Here's how the part is built. I have some questions about the finished solid (model axes, mm). Face numbers are marked on the shaded views. A direction names the side the tool comes from. Coordinates: 2 decimals unless noted, no trailing zeros. Write each loop counter-clockwise with the first axis right and the second up, starting at its lowest first coordinate (ties: lowest second). Pieces come first, ordered by that corner, then holes.
Item 1: For the marked faces 1 and 2, which set-ups out of +Z, -Z, +X, -X, +Y, -Y let a thin tool reach every point of the face, with its end or its side?
Item 2: If I drill on line 1 (Z direction, x = -0.05, y = -0.2); line 2 (Z direction, x = -0.85, y = -0.7); line 3 (X direction, y = -0.05, z = -7.75), over which ranges is the centre line in solid material (lowest first)?
Item 3: If we section it at A-A (z = -4.5): Please give me the cut outline in (x, y), then the cut area to 3 significant figures.
Item 4: I'm going to push flat-ended pins straight in: pin 1 Ø0.9 at (x, z) = (-0.5, -0.5) entering from -Y; pin 2 Ø0.9 at (x, z) = (0.5, -1) entering from -Y; pin 3 Ø1.3 at (y, z) = (1, -0.5) entering from -X; pin 4 Ø1.5 at (x, z) = (0.5, -6.5) entering from +Y. Where does each tip first touch, or does it pass through?
Autodesk Inventor part; units mm, degrees
ref_plane "MSC_PF1" through (0, 0, 0) normal (1, 0, 0) x (0, 1, 0)
ref_plane "MSC_PT1" through (0, 0, 0) normal (0, 0, -1) x (-1, 0, 0)
ref_plane "YZ Plane" through (0, 0, 0) normal (1, 0, 0) x (0, 1, 0)
sketch "Skizze1" plane through (0, 0, 0) normal (0, 1, 0) x (-1, 0, 0)
  point P0 (0, 0)
sketch "Skizze2" plane through (0, 0, 0) normal (0, 0, 1) x (1, 0, 0)
  point P0 (0, 0)
sketch "Skizze3" plane through (0, 0, 0) normal (0, 1, 0) x (-1, 0, 0)
  line L0 (-2.35, 0) -> (0, 0)
  line L1 (-2.35, -0.4) -> (-2.35, 0)
  line L2 (-1.25, -1.5) -> (-2.35, -0.4)
  line L3 (-1.25, -1.95) -> (-1.25, -1.5)
  line L4 (-1.025, -2.175) -> (-1.25, -1.95)
  line L5 (-1.25, -2.625) -> (-1.025, -2.175)
  line L6 (-1.25, -10) -> (-1.25, -2.625)
  line L7 (0, 0) -> (0, -10)
  line L8 (0, 3.3392) -> (0, -10.6608) construction
  line L9 (0, 3.3392) -> (0, -10.6608)
  line L10 (0, -13.4608) -> (0, 6.1392)
  line L11 (-1.25, -10) -> (0, -10)
  line L12 (0.47, 0) -> (-2.82, 0)
  dimension "d3" = 2.35
  dimension "d5" = 0.45
  dimension "d7" = 0.225
  dimension "d9" = 0.45
  dimension "d11" = 1.5
  dimension "d13" = 135
  dimension "d15" = 10
  dimension "d17" = 1.025
  dimension "d19" = 0
  dimension "d41" = 1.25
revolve "Drehung1" add sketch "Skizze3" angle 360 about axis through (0, 0, 3.3392) along (0, 0, -1)
sketch "Skizze4" plane through (0, 0, 0) normal (0, 1, 0) x (-1, 0, 0)
  line L0 (-1.4, 0) -> (0, 0)
  line L1 (-0.2333, -1.3636) -> (-1.4, 0)
  line L2 (0, -1.3636) -> (-0.2333, -1.3636)
  line L3 (0, 0) -> (0, -1.3636)
  line L4 (-1.25, -1.5) -> (1.25, -1.5) construction
  line L5 (-2.35, 0) -> (2.35, 0)
  line L6 (0, -1.8) -> (0, 0.3)
  dimension "d22" = 1.4
  dimension "d24" = 0.2333
  dimension "d26" = 1.3636
extrude "Extrusion1" cut sketch "Skizze4" along normal mid plane 0.4667
pattern_circular "Polare Anordnung1" count 4 over 360 about axis through (0, 0, 0) along (0, 0, 1) of "Extrusion1"
thread "Gewinde1"
ref_plane "MSC_PF1" through (0, 0, 0) normal (1, 0, 0) x (0, 1, 0)
ref_plane "MSC_PT1" through (0, 0, 0) normal (0, 0, -1) x (-1, 0, 0)
equation "\"d3\" = 0.5 * Dh"
equation "\"d5\" = msp_x"
equation "\"d7\" = ParA"
equation "\"d9\" = msp_x"
equation "\"d11\" = ParK"
equation "\"d15\" = NLG"
equation "\"d17\" = 0.5 * msp_mdtds"
equation "\"d41\" = 0.5 * NND"
equation "\"d22\" = 0.5 * M"
equation "\"d24\" = 0.0833333 * M"
equation "\"d26\" = 0.909091 * ParK"
equation "\"d27\" = 0.166667 * M"
equation "\"r\" = 0.6"
equation "\"PTC\" = 0.45"
equation "\"NLG\" = 10"
equation "\"ParK\" = 1.5"
equation "\"NND\" = 2.5"
equation "\"M\" = 2.8"
equation "\"Dh\" = 4.7"
equation "\"msp_c0\" = 4"
equation "\"msp_x\" = PTC"
equation "\"ParA\" = 0.5 * PTC"
equation "\"msp_mdtds\" = NND - PTC"
equation "\"THREADDIA\" = NND"
equation "\"TEMPLATE\" = 1.2345"
properties part number "DIN EN ISO 7046-2 Z - M2.5x10 - 8.8 - Z1" material "Stahl"
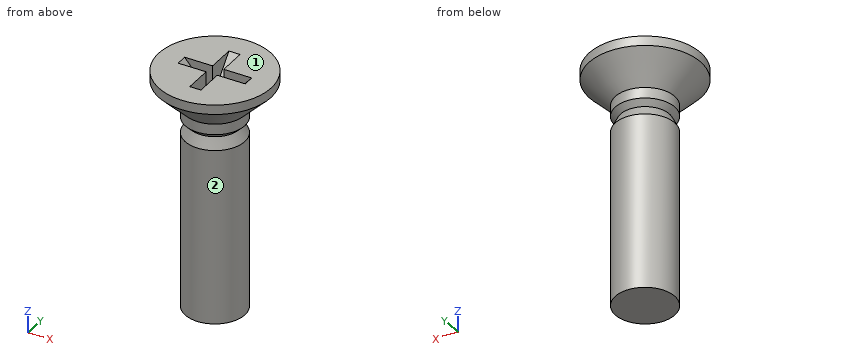
Answer list:
1. face 1: +Z, +X, -X, +Y, -Y
1. face 2: -Z
2. line 1: z = -10 to -1.36
2. line 2: z = -10 to -2.33, -2.1 to 0
2. line 3: x = -1.25 to 1.25
3. outline: circle Ø2.5 at (0, 0)
3. area: 4.91 mm2
4. pin 1: stops at y = -2.35
4. pin 2: stops at y = -2.15
4. pin 3: stops at x = -2.32
4. pin 4: stops at y = 1.25
